For this review, take the finished solid that the model builds, in its own axes (mm). A direction names the side the tool comes from. Coordinates: 2 decimals unless noted, no trailing zeros. Write each loop counter-clockwise with the first axis right and the second up, starting at its lowest first coordinate (ties: lowest second). Pieces come first, ordered by that corner, then holes. Notation, with made-up numbers: (-11.5, -6) - (19.5, -6) arc R7 cw to (19.5, 5) - close; hole circle Ø1 at (-35, 75). An arc over 180 degrees is marked (long way). Write each question's results on one line, items separated by ' | '.
from build123d import *

# Parameters (mm, degrees)
F0_W     = 102.648225
F0_H     = 51.967123
F1_DEPTH = 25.4
F2_R     = 6.35
F3_W     = 89.948225
F3_H     = 39.267123
F4_DEPTH = 19.05
F6_D     = 6.35
F6_DEPTH = 12.7


with BuildPart() as f1:
    # F0 (on Top) → F1 (new body)
    with BuildSketch(Plane.XY):
        with Locations((2.532753, 1.564751)):
            Rectangle(F0_W, F0_H)
    extrude(amount=F1_DEPTH)

    # F2
    f2_edges = [f1.edges().sort_by_distance(p)[0] for p in [
        (-48.79136, -24.41881, 12.7),
        (-48.79136, 27.548313, 12.7),
        (53.856865, -24.41881, 12.7),
        (53.856865, 27.548313, 12.7),
    ]]
    fillet(f2_edges, radius=F2_R)

    # F3 (on face) → F4 (cut)
    with BuildSketch(Plane.XY.offset(25.4)):
        with Locations((2.532753, 1.564751)):
            Rectangle(F3_W, F3_H)
    extrude(amount=-F4_DEPTH, mode=Mode.SUBTRACT)

    # F6
    with Locations(Plane(origin=(-48.79136, 0, 0), x_dir=(0, -1, 0), z_dir=(-1, 0, 0))):
        with Locations((0, 12.951535)):
            Hole(F6_D / 2, depth=F6_DEPTH)


solid = f1.part
Q1. Wall thickness on line 1 along Y through (x, z) = (-36.5, 8); line 2 along X through (y, z) = (4, 13.5); line 3 along Z through (x, y) = (-46.5, 0): over which ranges is each line inside the solid? List them lowest first. Write a range as from..to.
Results found:
line 1: -24.42..-18.07, 21.2..27.55 | line 2: -48.79..-42.44, 47.51..53.86 | line 3: 0..9.78, 16.13..25.4
Q2. For pin 1 (10 mm diameter, centred on y = -18.5, z = 15.5, fed in from -X); pin 2 (12 mm diameter, centred on x = -15, y = 7.5, fed in from +Z), all flat-tipped, find the tip position at first contact; note any pin that passes through.
Results found:
pin 1: x = -48.79 | pin 2: z = 6.35
Q3. Take a section at B-B on z = 19.5. State the section outline as (x, y) points.
Results found:
outline: (-48.79, -18.07) arc R6.35 ccw to (-42.44, -24.42) - (47.51, -24.42) arc R6.35 ccw to (53.86, -18.07) - (53.86, 21.2) arc R6.35 ccw to (47.51, 27.55) - (-42.44, 27.55) arc R6.35 ccw to (-48.79, 21.2) - close; hole (-42.44, -18.07) - (47.51, -18.07) - (47.51, 21.2) - (-42.44, 21.2) - close
Q4. Mouldability with a two-part tool opening along X and no side actions: class faces 1 (the face through (2, 2, 6.35)), 2 (the face through (2, 2, 0)), 3 (the face through (-48.791, 1.3, 9.7)) as pulls with the +X half, pulls with the -X half, needs draft (parallel to the pull), parting line crosses it, or undercut.
Results found:
face 1: undercut | face 2: needs draft | face 3: pulls with the -X half
Q5. Take a section at A-A on y = 0. State the section outline as (x, z) points, plus the area to 3 significant figures.
Results found:
outline: (-48.79, 0) - (53.86, 0) - (53.86, 25.4) - (47.51, 25.4) - (47.51, 6.35) - (-42.44, 6.35) - (-42.44, 9.78) - (-48.79, 9.78) - close; (-48.79, 16.13) - (-42.44, 16.13) - (-42.44, 25.4) - (-48.79, 25.4) - close | area: 853 mm2
Q6. Take a section at D-D on x = 7. State the section outline as (y, z) points.
Results found:
outline: (-24.42, 0) - (27.55, 0) - (27.55, 25.4) - (21.2, 25.4) - (21.2, 6.35) - (-18.07, 6.35) - (-18.07, 25.4) - (-24.42, 25.4) - close
Q7. For faces 4 (the face through (-45.572, 1.465, 10.135)), 5 (the face through (-42.441, 1, 18)), 6 (the face through (-46.98, 25.64, 12.88)), list the 3-axis set-ups (+Z, -Z, +X, -X, +Y, -Y) from which the entire face can be reached by the end or side of a thin tool; tool diameter is ignored.
Results found:
face 4: -X | face 5: +Z | face 6: +Z, -Z, -X, +Y
Q8. Take a section at C-C on y = 17.5. State the section outline as (x, z) points.
Results found:
outline: (-48.79, 0) - (53.86, 0) - (53.86, 25.4) - (47.51, 25.4) - (47.51, 6.35) - (-42.44, 6.35) - (-42.44, 25.4) - (-48.79, 25.4) - close
